Solid Edge part; units mm, degrees
sketch "Sketch1" plane through (0, 0, 0) normal (0, -1, 0) x (1, 0, 0)
  line L0 (75, -42) -> (75, 42)
  line L1 (75, 42) -> (-75, 42)
  line L2 (-75, 42) -> (-75, -42)
  line L3 (-75, -42) -> (75, -42)
extrude "Protrusion1" add sketch "Sketch1" along normal blind 2
sketch "Sketch2" plane through (0, 0, 0) normal (0, -1, 0) x (1, 0, 0)
  line L0 (-55, 38) -> (-55, 40)
  line L1 (-55, 40) -> (-65, 40)
  line L2 (-65, 40) -> (-65, 38)
  line L3 (-65, 38) -> (-55, 38)
  line L4 (-25, 40) -> (-35, 40)
  line L5 (-35, 40) -> (-35, 38)
  line L6 (-35, 38) -> (-25, 38)
  line L7 (-25, 38) -> (-25, 40)
  line L8 (-5, 38) -> (5, 38)
  line L9 (5, 38) -> (5, 40)
  line L10 (5, 40) -> (-5, 40)
  line L11 (-5, 40) -> (-5, 38)
  line L12 (25, 38) -> (35, 38)
  line L13 (35, 38) -> (35, 40)
  line L14 (35, 40) -> (25, 40)
  line L15 (25, 40) -> (25, 38)
  line L16 (55, 38) -> (65, 38)
  line L17 (65, 38) -> (65, 40)
  line L18 (65, 40) -> (55, 40)
  line L19 (55, 40) -> (55, 38)
  line L20 (65, -40) -> (65, -38)
  line L21 (65, -38) -> (55, -38)
  line L22 (55, -38) -> (55, -40)
  line L23 (55, -40) -> (65, -40)
  line L24 (25, -40) -> (35, -40)
  line L25 (35, -40) -> (35, -38)
  line L26 (35, -38) -> (25, -38)
  line L27 (25, -38) -> (25, -40)
  line L28 (5, -38) -> (-5, -38)
  line L29 (-5, -38) -> (-5, -40)
  line L30 (-5, -40) -> (5, -40)
  line L31 (5, -40) -> (5, -38)
  line L32 (-25, -38) -> (-35, -38)
  line L33 (-35, -38) -> (-35, -40)
  line L34 (-35, -40) -> (-25, -40)
  line L35 (-25, -40) -> (-25, -38)
  line L36 (-55, -40) -> (-55, -38)
  line L37 (-55, -38) -> (-65, -38)
  line L38 (-65, -38) -> (-65, -40)
  line L39 (-65, -40) -> (-55, -40)
  line L40 (-73, -42) -> (-73, -25)
  line L41 (-73, -25) -> (-75, -25)
  line L42 (-75, -25) -> (-75, -42)
  line L43 (-75, -42) -> (-73, -42)
  line L44 (-73, -15) -> (-73, -5)
  line L45 (-73, -5) -> (-75, -5)
  line L46 (-75, -5) -> (-75, -15)
  line L47 (-75, -15) -> (-73, -15)
  line L48 (-73, 5) -> (-73, 15)
  line L49 (-73, 15) -> (-75, 15)
  line L50 (-75, 15) -> (-75, 5)
  line L51 (-75, 5) -> (-73, 5)
  line L52 (-73, 25) -> (-73, 42)
  line L53 (-73, 42) -> (-75, 42)
  line L54 (-75, 42) -> (-75, 25)
  line L55 (-75, 25) -> (-73, 25)
  line L56 (75, 25) -> (75, 42)
  line L57 (75, 42) -> (73, 42)
  line L58 (73, 42) -> (73, 25)
  line L59 (73, 25) -> (75, 25)
  line L60 (73, 15) -> (73, 5)
  line L61 (73, 5) -> (75, 5)
  line L62 (75, 5) -> (75, 15)
  line L63 (75, 15) -> (73, 15)
  line L64 (73, -5) -> (73, -15)
  line L65 (73, -15) -> (75, -15)
  line L66 (75, -15) -> (75, -5)
  line L67 (75, -5) -> (73, -5)
  line L68 (73, -25) -> (73, -42)
  line L69 (73, -42) -> (75, -42)
  line L70 (75, -42) -> (75, -25)
  line L71 (75, -25) -> (73, -25)
extrude "ExtrudedCutout_1" cut sketch "Sketch2" along normal blind 2
fillet "Round_1" radius 1 4 edges at (-73, -1, -42) (73, -1, -42) (73, -1, 42) (-73, -1, 42)
properties material "Acrylic, high impact grade"
For this review, take the finished solid that the model builds, in its own axes (mm). Round coordinates to 2 decimals unless told otherwise and drop trailing zeros. Order: outer loops, then holes, each group sorted by start corner. A loop starts at its lowest first (then second) coordinate and runs counter-clockwise, first axis right, second up. Notation, with made-up numbers: (81, 13.5) -> (140, 13.5) arc R28 cw to (140, 50.5) -> close; hole circle Ø5 at (40.5, 61). An arc over 180 degrees is marked (long way). Use a Markdown table: item, result.
Item 1: Take a section at A-A (x = 1.5). State the section outline as (y, z) points.
Resolved:
| item | result |
|---|---|
| outline | (-2, -42) -> (0, -42) -> (0, -40) -> (-2, -40) -> close; (-2, -38) -> (0, -38) -> (0, 38) -> (-2, 38) -> close; (-2, 40) -> (0, 40) -> (0, 42) -> (-2, 42) -> close |
Item 2: For line 1 along Z through (x, y) = (-62, -0.3); line 2 along X through (y, z) = (-0.9, 38.5); line 3 along X through (y, z) = (-1.35, -13), list the stretches that pass through material, from the lowest coordinate up. Write a range as [from, to].
Resolved:
| item | result |
|---|---|
| line 1 | z = [-42, -40], [-38, 38], [40, 42] |
| line 2 | x = [-73, -65], [-55, -35], [-25, -5], [5, 25], [35, 55], [65, 73] |
| line 3 | x = [-73, 73] |
Item 3: Take a section at B-B (y = -1.15). State how many separate pieces and enclosed holes the cut face has, plus the area to 3 significant figures.
Resolved:
| item | result |
|---|---|
| separate pieces | 1 |
| enclosed holes | 10 |
| area | 12,200 mm² |
Item 4: Take a section at C-C (z = 11.5). State the section outline as (x, y) points, plus the area to 3 significant figures.
Resolved:
| item | result |
|---|---|
| outline | (-73, -2) -> (73, -2) -> (73, 0) -> (-73, 0) -> close |
| area | 292 mm² |
Item 5: For pin 1 (0.6 mm diameter, centred on x = 74.5, y = -0.5, fed in from +Z); pin 2 (1 mm diameter, centred on y = -0.5, z = 39, fed in from -X); pin 3 (12 mm diameter, centred on x = 28, z = 3, fed in from +Y), all flat-tipped, find the tip position at first contact; note any pin that passes through.
Resolved:
| item | result |
|---|---|
| pin 1 | stops at z = 25 |
| pin 2 | stops at x = -73 |
| pin 3 | stops at y = 0 |
